```python
from build123d import *

# Parameters (mm, degrees)
F0_R     = 9.525
F1_DEPTH = 3.175


with BuildPart() as f1:
    # F0 (on Front) → F1 (new body)
    with BuildSketch(Plane.XZ):
        with BuildLine():
            Line((-6.35, 12.7), (-12.7, 12.7))
            ThreePointArc((-12.7, 12.7), (-19.05, 0), (-12.7, -12.7))
            Line((-12.7, -12.7), (-6.35, -12.7))
            Line((-6.35, -12.7), (-6.35, -15.875))
            Line((-6.35, -15.875), (6.35, -15.875))
            Line((6.35, -15.875), (6.35, -12.7))
            Line((6.35, -12.7), (12.7, -12.7))
            ThreePointArc((12.7, -12.7), (19.05, 0), (12.7, 12.7))
            Line((12.7, 12.7), (6.35, 12.7))
            Line((6.35, 12.7), (6.35, 15.875))
            Line((6.35, 15.875), (-6.35, 15.875))
            Line((-6.35, 15.875), (-6.35, 12.7))
        make_face()
        Circle(F0_R, mode=Mode.SUBTRACT)
    extrude(amount=F1_DEPTH)


solid = f1.part
```
Read the model definition and answer for the solid it produces. Units are mm, in the model's axes. A direction names the side the tool comes from. Coordinates: 2 decimals unless noted, no trailing zeros. Write each loop counter-clockwise with the first axis right and the second up, starting at its lowest first coordinate (ties: lowest second). Pieces come first, ordered by that corner, then holes. Notation, with made-up numbers: (32, -2.75) - (57, -2.75) arc R24 cw to (57, 23.25) - close; hole circle Ø7 at (84, 49). An arc over 180 degrees is marked (long way). Answer as a JSON object with one key per item and string values. Group by question number.
1. The mould has two halves that part along Z. Classify faces 6 (the cylindrical face through (-7.559, -1.565, -5.796)), 7 (the flat face through (10, -2, 12.7)), 8 (the flat face through (-6.35, -2, -14)): +Z half, -Z half, draft (parallel to the pull), parting line (faces both ways), or undercut.
2. A cutting plane is placed at A-A (y = -0.9). Determine the outline of the cut face in (x, z) (3 decimals).
3. Which of the six approach directions +Z, -Z, +X, -X, +Y, -Y give full straight-line access (tool end or side, diameter ignored) to faces 1 (the flat face through (-9, -2, 12.7)), 2 (the flat face through (-10, -2, -12.7)), 3 (the flat face through (6.35, -2, -14)), 4 (the flat face through (6.35, -2, 14)), 5 (the cylindrical face through (19.05, -1.57, -0.21))?
4. A cutting plane is placed at C-C (x = -8.5). Determine the outline of the cut face in (y, z) (3 decimals).
5. A cutting plane is placed at B-B (z = 0). Determine the outline of the cut face in (x, y) (3 decimals), plus the area to 3 significant figures.
6. Each of these flat-tipped pins is pushed along its axis until it touches: P1, Ø1.6, axis at x = 10, y = -1.5, coming from the -Z side; P2, Ø1.6, axis at x = -9.5, y = -1.5, coming from the +Z side; P3, Ø1.6, axis at y = -1.5, z = 14, coming from the -X side. Where does it stop, or does it pass through?
7. Consider L1, parallel to Z at x = 0, y = -2 (3 decimals); L2, parallel to Z at x = -12, y = -0.85; L3, parallel to Z at x = 2, y = -2.45 (3 decimals). Determine where each line is inside the solid, lowest interval first. Write a range as [from, to].
Worked out:
{
 "1": {"face 6": "undercut", "face 7": "+Z half", "face 8": "draft"},
 "2": {"outline": "(-12.7, -12.7) - (-6.35, -12.7) - (-6.35, -15.875) - (6.35, -15.875) - (6.35, -12.7) - (12.7, -12.7) arc R15.875 ccw to (12.7, 12.7) - (6.35, 12.7) - (6.35, 15.875) - (-6.35, 15.875) - (-6.35, 12.7) - (-12.7, 12.7) arc R15.875 ccw to start; hole circle Ø19.05 at (0, 0)"},
 "3": {"face 1": "+Z, -X, +Y, -Y", "face 2": "-Z, -X, +Y, -Y", "face 3": "-Z, +X, +Y, -Y", "face 4": "+Z, +X, +Y, -Y", "face 5": "+X, +Y, -Y"},
 "4": {"outline": "(-3.175, -12.7) - (0, -12.7) - (0, -4.298) - (-3.175, -4.298) - close; (-3.175, 4.298) - (0, 4.298) - (0, 12.7) - (-3.175, 12.7) - close"},
 "5": {"outline": "(-19.05, -3.175) - (-9.525, -3.175) - (-9.525, 0) - (-19.05, 0) - close; (9.525, -3.175) - (19.05, -3.175) - (19.05, 0) - (9.525, 0) - close", "area": "60.5 mm²"},
 "6": {"P1": "stops at z = -12.7", "P2": "stops at z = 12.7", "P3": "stops at x = -6.35"},
 "7": {"L1": "z = [-15.875, -9.525], [9.525, 15.875]", "L2": "z = [-12.7, 12.7]", "L3": "z = [-15.875, -9.313], [9.313, 15.875]"}
}
